Work out the finished part from the listing and answer in its coordinate system (mm). Give positions to 0.01 mm unless a question says otherwise; leave off trailing zeros. Loops run counter-clockwise (first coordinate to the right, second up) from the corner with the lowest first, then second, coordinate; pieces in that order, holes last. Notation, with made-up numbers: M 23.25,13 L 62.25,13 A17 ccw 62.25,28 Z; hole C 7.5,64.5 d5. An arc over 180 degrees is marked long. Write item = value, one per line. Start each with the question number.
1. Section A-A on y = -0.6 is taken. Determine the outline of the cut face in (x, z), plus the area to 3 significant figures.
2. The mould has two halves that part along X. Classify faces 1 (the face through (-8, -1, -11)), 2 (the face through (12.7, -0.5, 12.3)), 3 (the face through (-12.7, -0.5, -12.3)), 4 (the face through (-2.75, -0.49, -12.38)): released by +X, released by -X, zero draft, split by the parting line, or undercut.
3. Section D-D on z = -2.5 is taken. Determine the outline of the cut face in (x, y).
4. Consider L1, parallel to Z at x = 8.5, y = -0.1; L2, parallel to Z at x = 1, y = -0.2; L3, parallel to X at y = -0.4, z = -4. Determine where each line is inside the solid, lowest interval first. Write a range as [from, to].
5. Section C-C on x = 14 is taken. Determine the outline of the cut face in (y, z).
6. Section B-B on z = 10 is taken. Determine the outline of the cut face in (x, y), plus the area to 3 significant figures.
```python
from build123d import *

# Parameters (mm, degrees)
F0_R     = 12.679986
F1_DEPTH = 1


with BuildPart() as f1:
    # F0 (on Front) → F1 (new body)
    with BuildSketch(Plane.XZ):
        Polygon((0, 25), (-25, 0), (0, -25), (25, 0), align=None)
        Circle(F0_R, mode=Mode.SUBTRACT)
    extrude(amount=F1_DEPTH)


solid = f1.part
```
Verdict:
q1.outline = M -25,0 L 0,-25 L 25,0 L 0,25 Z; hole C 0,0 d25.36
q1.area = 745 mm2
q2.face_1 = zero draft
q2.face_2 = released by +X
q2.face_3 = released by -X
q2.face_4 = undercut
q3.outline = M -22.5,-1 L -12.43,-1 L -12.43,0 L -22.5,0 Z; M 12.43,-1 L 22.5,-1 L 22.5,0 L 12.43,0 Z
q4.L1 = [-16.5, -9.41], [9.41, 16.5]
q4.L2 = [-24, -12.64], [12.64, 24]
q4.L3 = [-21, -12.03], [12.03, 21]
q5.outline = M -1,-11 L 0,-11 L 0,11 L -1,11 Z
q6.outline = M -15,-1 L -7.8,-1 L -7.8,0 L -15,0 Z; M 7.8,-1 L 15,-1 L 15,0 L 7.8,0 Z
q6.area = 14.4 mm2
